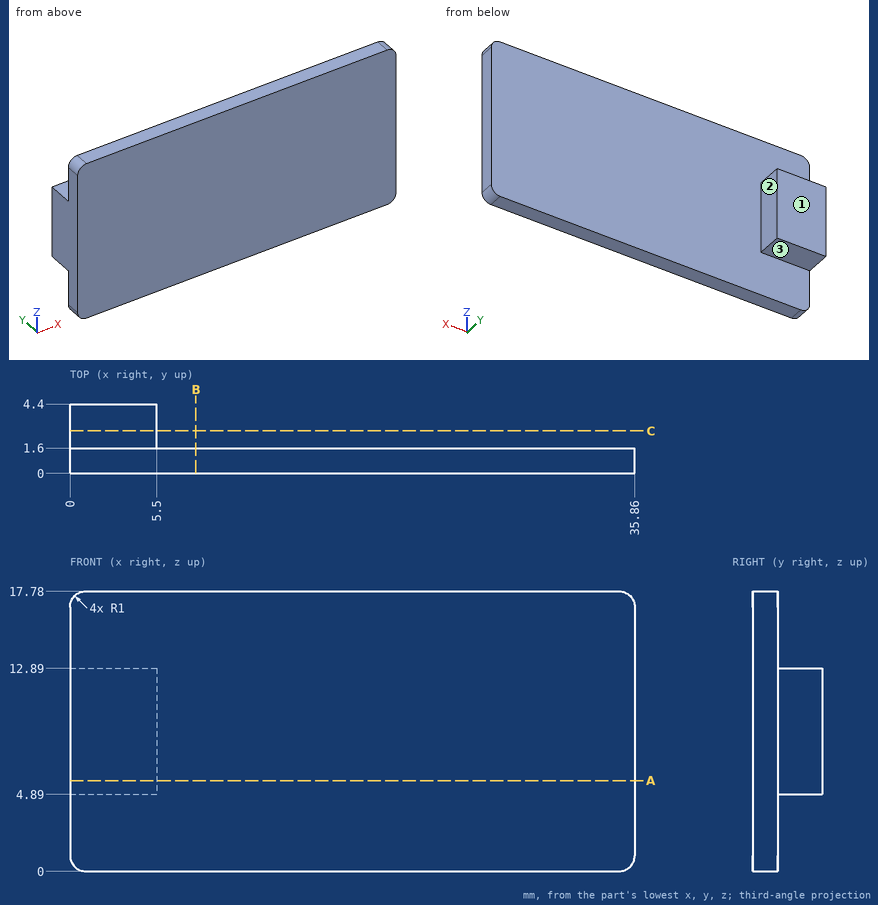
Here's the drawing with two shaded views (mm, measured from the low corner). I have some questions. A direction names the side the tool comes from. Give positions to 0.01 mm unless a question says otherwise; leave off trailing zeros. Order: outer loops, then holes, each group sorted by start corner. A loop starts at its lowest first (then second) coordinate and runs counter-clockwise, first axis right, second up.
Q1. Suppose I cut it at B-B, the plane x = 8. Write out the boundary of the cut face in (y, z), and give its area (3 significant figures).
Q2. Suppose I cut it at A-A, the plane z = 5.75. Write out the boundary of the cut face in (x, y), and give its area (3 significant figures).
Q3. For the marked faces 1, 2 and 3, which set-ups out of +Z, -Z, +X, -X, +Y, -Y let a thin tool reach every point of the face, with its end or its side?
Q4. If I drill on line 1 along Y through (x, z) = (13.5, 5.75); line 2 along X through (y, z) = (3.65, 5); line 3 along Z through (x, y) = (3.5, 2.3), over which ranges is the centre line in solid material (lowest first)?
Q5. I'm going to push flat-ended pins straight in: P1, Ø4, axis at x = 21, z = 14, coming from the +Y side; P2, Ø0.8, axis at x = 2.5, y = 3.5, coming from the +Z side. Where does each tip first touch, or does it pass through?
Q6. Suppose I cut it at C-C, the plane y = 2.7. Write out the boundary of the cut face in (x, z).
Solution:
1. outline: (0, 0) - (1.6, 0) - (1.6, 17.78) - (0, 17.78) - close
1. area: 28.4 mm2
2. outline: (0, 0) - (35.86, 0) - (35.86, 1.6) - (5.5, 1.6) - (5.5, 4.4) - (0, 4.4) - close
2. area: 72.8 mm2
3. face 1: +Z, -Z, +X, -X, +Y
3. face 2: +Z, -Z, +X, +Y
3. face 3: -Z, +X, -X, +Y
4. line 1: y = 0 to 1.6
4. line 2: x = 0 to 5.5
4. line 3: z = 4.89 to 12.89
5. P1: stops at y = 1.6
5. P2: stops at z = 12.89
6. outline: (0, 4.89) - (5.5, 4.89) - (5.5, 12.89) - (0, 12.89) - close
